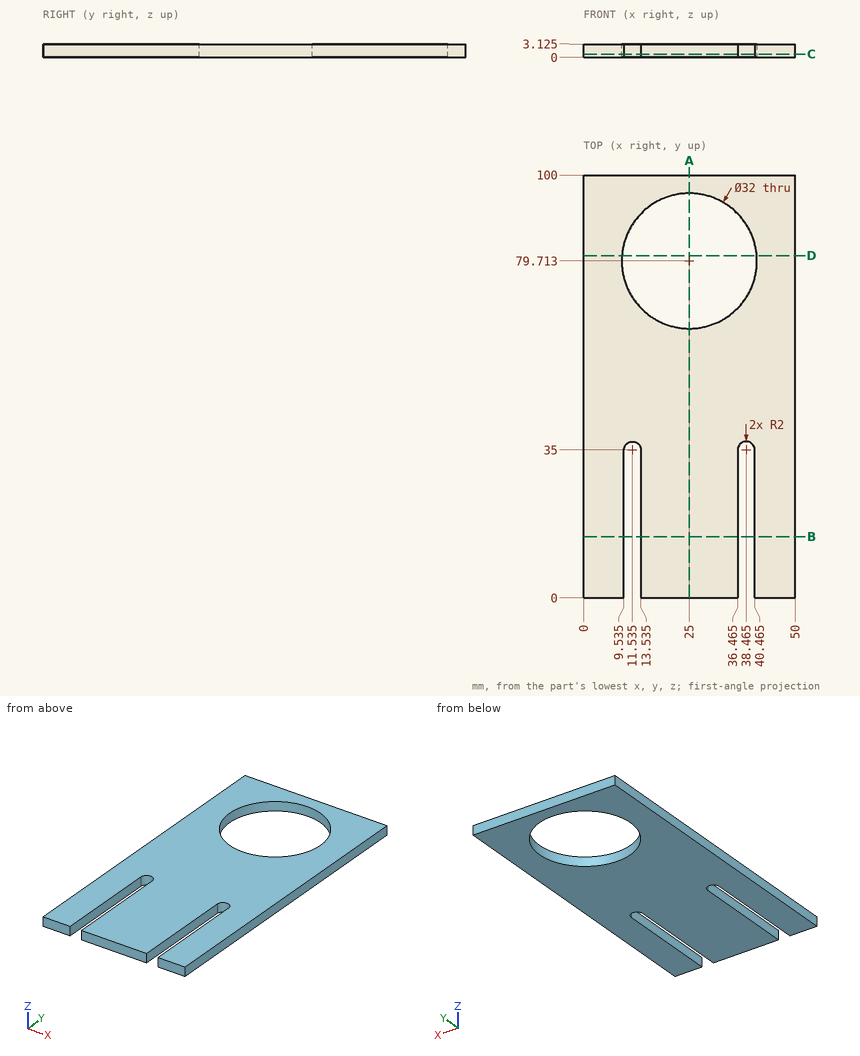
Can you work these out from the drawing? Everything is in mm from the part's minimum corner. Give positions to 0.01 mm unless a question says otherwise; leave off trailing zeros. Write each loop counter-clockwise with the first axis right and the second up, starting at its lowest first coordinate (ties: lowest second). Pieces come first, ordered by that corner, then holes. Notation, with made-up numbers: M 68,83 L 119,83 A31 cw 119,113 Z; hole C 56.5,81 d1. An arc over 180 degrees is marked long. Answer in a Markdown table with one row per item. Add a question column.
Item 1: Imagine slicing it at D-D, the plane y = 81. Write out the boundary of the cut face in (x, z) (1 decimal).
Item 2: Imagine slicing it at A-A, the plane x = 25. Write out the boundary of the cut face in (y, z) (1 decimal).
Item 3: For pin 1 Ø1.5 at (x, y) = (30.5, 35.5) entering from -Z, with a flat end and sliding along its axis, tell me the tip position at first contact or that it passes through.
Item 4: Imagine slicing it at B-B, the plane y = 14.5. Write out the boundary of the cut face in (x, z) (1 decimal).
Item 5: Please list where these lines run through material, in increasing order: L1, parallel to X at y = 19.5, z = 2.65 (1 decimal); L2, parallel to Y at x = 25, z = 1; L3, parallel to X at y = 79, z = 1.6.
Item 6: Imagine slicing it at C-C, the plane z = 0.7. Write out the boundary of the cut face in (x, y) (1 decimal).
Evaluation:
| question | item | result |
|---|---|---|
| 1 | outline | M 0,0 L 9.1,0 L 9.1,3.1 L 0,3.1 Z; M 40.9,0 L 50,0 L 50,3.1 L 40.9,3.1 Z |
| 2 | outline | M 0,0 L 63.7,0 L 63.7,3.1 L 0,3.1 Z; M 95.7,0 L 100,0 L 100,3.1 L 95.7,3.1 Z |
| 3 | pin 1 | stops at z = 0 |
| 4 | outline | M 0,0 L 9.5,0 L 9.5,3.1 L 0,3.1 Z; M 13.5,0 L 36.5,0 L 36.5,3.1 L 13.5,3.1 Z; M 40.5,0 L 50,0 L 50,3.1 L 40.5,3.1 Z |
| 5 | L1 | x = 0 to 9.5, 13.5 to 36.5, 40.5 to 50 |
| 5 | L2 | y = 0 to 63.71, 95.71 to 100 |
| 5 | L3 | x = 0 to 9.02, 40.98 to 50 |
| 6 | outline | M 0,0 L 9.5,0 L 9.5,35 A2 cw 13.5,35 L 13.5,0 L 36.5,0 L 36.5,35 A2 cw 40.5,35 L 40.5,0 L 50,0 L 50,100 L 0,100 Z; hole C 25,79.7 d32 |
